Read the model definition and answer for the solid it produces. Units are mm, in the model's axes. A direction names the side the tool comes from. Round coordinates to 2 decimals unless told otherwise and drop trailing zeros. Order: outer loops, then holes, each group sorted by start corner. A loop starts at its lowest first (then second) coordinate and runs counter-clockwise, first axis right, second up.
from build123d import *

# Parameters (mm, degrees)
EXTRUDE_1_DEPTH     = 18
EXTRUDE_2_DEPTH     = 4
CUT_EXTRUDE_1_DEPTH = 7
SKETCH_4_W          = 2.5
SKETCH_4_H          = 7.5
EXTRUDE_3_DEPTH     = 2.5


with BuildPart() as part:
    # Эскиз1 → Бобышка-Вытянуть1 (new body, symmetric)
    with BuildSketch(Plane.XY):
        Polygon((0, 78), (0, 0), (78, 0), (78, 6), (6, 6), (6, 78), align=None)
    extrude(amount=EXTRUDE_1_DEPTH, both=True)

    # Эскиз2 → Бобышка-Вытянуть2 (add)
    with BuildSketch(Plane.XY.offset(18)):
        Polygon((78, 6), (6, 6), (6, 78), (12, 78), (78, 12), align=None)
    extrude(amount=-EXTRUDE_2_DEPTH)

    # Эскиз3 → Вырез-Вытянуть1 (cut, through all)
    with BuildSketch(Plane(origin=(0, 6, 0), x_dir=(1, 0, 0), z_dir=(0, 1, 0))):
        with BuildLine():
            Line((18, 4.3), (31.4, 4.3))
            ThreePointArc((31.4, 4.3), (35.7, 0), (31.4, -4.3))
            Line((31.4, -4.3), (18, -4.3))
            ThreePointArc((18, -4.3), (13.7, 0), (18, 4.3))
        make_face()
        with BuildLine():
            Line((56.4, 4.3), (60, 4.3))
            ThreePointArc((60, 4.3), (64.3, 0), (60, -4.3))
            Line((60, -4.3), (56.4, -4.3))
            ThreePointArc((56.4, -4.3), (52.1, 0), (56.4, 4.3))
        make_face()
    cut_extrude_1 = extrude(amount=-CUT_EXTRUDE_1_DEPTH, mode=Mode.SUBTRACT)

    # Эскиз4 → Бобышка-Вытянуть3 (add)
    with BuildSketch(Plane.XZ):
        with Locations((4.25, 0)):
            Rectangle(SKETCH_4_W, SKETCH_4_H)
        with Locations((73.75, 0)):
            Rectangle(SKETCH_4_W, SKETCH_4_H)
    extrude_3 = extrude(amount=EXTRUDE_3_DEPTH)

    # Зеркальное отражение3: Вырез-Вытянуть1, Бобышка-Вытянуть3 across plane
    add(cut_extrude_1.mirror(Plane(origin=(0, 0, 0), x_dir=(0, 0, 1), z_dir=(-0.707106781, 0.707106781, 0))), mode=Mode.SUBTRACT)
    add(extrude_3.mirror(Plane(origin=(0, 0, 0), x_dir=(0, 0, 1), z_dir=(-0.707106781, 0.707106781, 0))))


solid = part.part
Q1. For a pull along Z with two mould halves and no side action, classify faces 4 (the face through (31, 31, 18)), 5 (the face through (38, 0, 0)), 6 (the face through (64.3, 3, -0.1)) as released by +Z, released by -Z, zero draft, split by the parting line, or undercut.
Outcome:
face 4: released by +Z
face 5: zero draft
face 6: undercut
Q2. For faces 1 (the face through (-1, 74, -3.75)), 2 (the face through (3, 25, 4.3)), 3 (the face through (58, 3, 4.3)), determine the directions among +Z, -Z, +X, -X, +Y, -Y from which every point of the face is accessible in a straight line to the end or side of a thin tool.
Outcome:
face 1: -Z, -X, +Y, -Y
face 2: +X, -X
face 3: +Y, -Y
Q3. A cutting plane is placed at B-B, the plane x = 51. Give the vertices of the cut face in (y, z).
Outcome:
outline: (0, -18) - (6, -18) - (6, 14) - (39, 14) - (39, 18) - (0, 18) - close
Q4. A cutting plane is placed at A-A, the plane y = 27. Give the vertices of the cut face in (x, z).
Outcome:
outline: (0, -18) - (6, -18) - (6, -4.3) - (0, -4.3) - close; (0, 4.3) - (6, 4.3) - (6, 14) - (63, 14) - (63, 18) - (0, 18) - close
Q5. Straight lines are drawn through the part: probe 1 along X at (y, z) = (8, -3); probe 2 along Z at (x, y) = (32, 8). For each, find the intervals that lie inside material, in ascending order.
Outcome:
probe 1: x = 0 to 6
probe 2: z = 14 to 18
Q6. Flat-ended cylindrical pins translate along their axes: pin 1 (0.8 mm diameter, centred on y = -1.5, z = 1, fed in from +X); pin 2 (18 mm diameter, centred on y = 29.5, z = -9, fed in from -X); pin 3 (5 mm diameter, centred on x = 70, z = 6.5, fed in from +Y). Find the tip coordinate at first contact, or state that the pin passes through.
Outcome:
pin 1: stops at x = 75
pin 2: stops at x = 0
pin 3: stops at y = 6
Q7. A cutting plane is placed at C-C, the plane z = 6. Give the vertices of the cut face in (x, y).
Outcome:
outline: (0, 0) - (78, 0) - (78, 6) - (6, 6) - (6, 78) - (0, 78) - close
Q8. A cutting plane is placed at D-D, the plane y = 58. Give the vertices of the cut face in (x, z), plus the area to 3 significant figures.
Outcome:
outline: (0, -18) - (6, -18) - (6, -4.3) - (0, -4.3) - close; (0, 4.3) - (6, 4.3) - (6, 14) - (32, 14) - (32, 18) - (0, 18) - close
area: 268 mm2
